Autodesk Inventor part; units mm, degrees
ref_plane "YZ Plane" through (0, 0, 0) normal (1, 0, 0) x (0, 1, 0)
ref_plane "XZ Plane" through (0, 0, 0) normal (0, 1, 0) x (-1, 0, 0)
ref_plane "XY Plane" through (0, 0, 0) normal (0, 0, 1) x (1, 0, 0)
sketch "Sketch1" plane through (0, 0, 0) normal (0, 0, 1) x (1, 0, 0)
  circle A0 centre (0, 0) radius 80
  dimension "d0" = 160
extrude "Extrusion1" add sketch "Sketch1" along normal blind 27.5
sketch "Sketch2" plane through (0, 0, 27.5) normal (0, 0, 1) x (1, 0, 0)
  circle A0 centre (0, 0) radius 70
  dimension "d3" = 140
extrude "Extrusion2" cut sketch "Sketch2" against normal blind 20
fillet "Fillet3" radius 12.5 1 edges at (-70, 0, 7.5)
fillet "Fillet4" radius 27.5 1 edges at (-80, 0, 0)
sketch "Sketch4" plane through (0, 0, 7.5) normal (0, 0, 1) x (1, 0, 0)
  circle A0 centre (0, 0) radius 21
  dimension "d13" = 42
extrude "Extrusion4" add sketch "Sketch4" along normal blind 8
sketch "Sketch6" plane through (0, 0, 27.5) normal (0, 0, 1) x (1, 0, 0)
  point P0 (0, 0)
  point P1 (0, 75)
  point P2 (75, 0)
  point P3 (0, -75)
  point P4 (-75, 0)
  dimension "d24" = 75
  dimension "d25" = 75
  dimension "d26" = 75
hole "Hole2" at (0, 75, 27.5) at (75, 0, 27.5) at (0, -75, 27.5) at (-75, 0, 27.5) direction (0, 0, -1) diameter 3.242 depth 10
sketch "Sketch8" plane through (0, 0, 15.5) normal (0, 0, 1) x (1, 0, 0)
  point P0 (0, 0)
  point P1 (0, 0)
hole "Hole4" at (0, 0, 15.5) direction (0, 0, -1) diameter 3.5 end through all
sketch "Sketch9" plane through (0, 0, 0) normal (0, 0, -1) x (-1, 0, 0)
  circle A0 centre (0, 0) radius 1.75
  circle A1 centre (0, 0) radius 19
  dimension "d56" = 38
extrude "Extrusion5" cut sketch "Sketch9" against normal blind 9
sketch "Sketch10" plane through (0, 0, 9) normal (0, 0, -1) x (-1, 0, 0)
  circle A0 centre (0, 0) radius 1.75
  circle A1 centre (0, 0) radius 6.75
  dimension "d59" = 13.5
extrude "Extrusion6" cut sketch "Sketch10" against normal blind 4.6
sketch "Sketch11" plane through (0, 0, 15.5) normal (0, 0, 1) x (1, 0, 0)
  point P0 (0, 0)
  point P1 (12.5, 0)
  point P2 (-12.5, 0)
  dimension "d74" = 12.5
  dimension "d75" = 12.5
hole "Hole5" at (12.5, 0, 15.5) at (-12.5, 0, 15.5) direction (0, 0, -1) diameter 3.2 end through all counterbore diameter 6 counterbore depth 3.2
sketch "Sketch13" plane through (0, 0, 7.5) normal (0, 0, 1) x (1, 0, 0)
  circle A0 centre (0, 0) radius 21
  line L0 (12.5, -16.8745) -> (12.5, -23.249)
  line L1 (12.5, -23.249) -> (-12.5, -23.249)
  line L2 (-12.5, -23.249) -> (-12.5, -16.8745)
  dimension "d88" = 25
  dimension "d89" = 12.5
extrude "Extrusion7" add sketch "Sketch13" along normal blind 8 contours A0 L0 L1 L2
sketch "Sketch18" plane through (0, 0, 15.5) normal (0, 0, 1) x (1, 0, 0)
  point P0 (0, 0)
  point P1 (11.3, -14.5)
  point P2 (-11.3, -14.5)
  dimension "d119" = 14.5
  dimension "d120" = 11.3
  dimension "d121" = 11.3
  dimension "d122" = 14.5
hole "Hole8" at (11.3, -14.5, 15.5) at (-11.3, -14.5, 15.5) direction (0, 0, -1) diameter 1.567 depth 5
sketch "Sketch20" plane through (0, 0, 15.5) normal (0, 0, 1) x (1, 0, 0)
  line L0 (9.25, -9.249) -> (-9.25, -9.249)
  line L1 (-9.25, -9.249) -> (-9.25, -20.249)
  line L2 (-9.25, -20.249) -> (9.25, -20.249)
  line L3 (9.25, -20.249) -> (9.25, -9.249)
  line L4 (-12.5, -23.249) -> (12.5, -23.249)
  circle A0 centre (11.3, -14.5) radius 0.7835
  point P0 (0, 0)
  dimension "d141" = 14
  dimension "d142" = 3
  dimension "d171" = 9.25
  dimension "d172" = 9.25
extrude "Extrusion12" cut sketch "Sketch20" against normal blind 17 contours L3 L2 L1 L0
fillet "Fillet10" radius 3 4 edges at (9.25, -9.249, 12.25) (9.25, -20.249, 7.75) (-9.25, -9.249, 12.25) (-9.25, -20.249, 7.75)
fillet "Fillet11" radius 3 4 edges at (12.5, -16.8745, 11.5) (12.5, -23.249, 11.5) (-12.5, -23.249, 11.5) (-12.5, -16.8745, 11.5)
chamfer "Chamfer2" distance 0.25 angle 45 4 edges at (0, 21, 15.5) (-12.5, -19.2862, 15.5) (0, -23.249, 15.5) (12.5, -19.2862, 15.5)
sketch "Sketch21" plane through (0, 0, 7.5) normal (0, 0, 1) x (1, 0, 0)
  circle A0 centre (0, 0) radius 1.75
  circle A1 centre (-40, -20) radius 4
  circle A2 centre (-40, 20) radius 4
  circle A3 centre (40, -20) radius 4
  circle A4 centre (40, 20) radius 4
  dimension "d147" = 40
  dimension "d148" = 20
  dimension "d149" = 20
  dimension "d150" = 20
  dimension "d151" = 20
  dimension "d152" = 40
  dimension "d153" = 40
  dimension "d154" = 40
  dimension "d155" = 8
  dimension "d156" = 8
  dimension "d157" = 8
  dimension "d158" = 8
extrude "Extrusion13" add sketch "Sketch21" along normal blind 3 contours A1 | A2 | A3 | A4
sketch "Sketch22" plane through (-40, 20, 10.5) normal (0, 0, 1) x (1, 0, 0)
  circle A0 centre (0, -40) radius 4
  circle A1 centre (80, 0) radius 4
  circle A2 centre (80, -40) radius 4
  point P0 (40, -20)
  point P1 (0, 0)
hole "Hole9" at (-40, -20, 10.5) at (-40, 20, 10.5) at (40, 20, 10.5) at (40, -20, 10.5) direction (0, 0, -1) diameter 3 end through all counterbore diameter 6 counterbore depth 3.2
chamfer "Chamfer3" distance 0.2 angle 45 19 edges at (36, -20, 10.5) (-44, -20, 10.5) (-44, 20, 10.5) (36, 20, 10.5) (-40, -17, 10.5) (40, -17, 10.5) (-40, 23, 10.5) (40, 23, 10.5) (8.3713, -10.1276, 15.5) (0, -9.249, 15.5) (-8.3713, -10.1276, 15.5) (-9.25, -14.749, 15.5) (-8.3713, -19.3703, 15.5) (0, -20.249, 15.5) (8.3713, -19.3703, 15.5) (9.25, -14.749, 15.5) (0, 1.75, 15.5) (-12.5, 3, 15.5) (12.5, 3, 15.5)
chamfer "Chamfer5" distance 1 angle 45 6 edges at (0, 19, 0) (0, -20.249, 0) (8.3713, -19.3703, 0) (9.25, -16.9226, 0) (-8.3713, -19.3703, 0) (-9.25, -16.9226, 0)
chamfer "Chamfer6" distance 0.5 angle 45 3 edges at (-70, 0, 27.5) (-80, 0, 27.4995) (-80, 0, 27.5)
properties part number "bottom cover" material "Aluminum 6061"
Work out the finished part from the listing and answer in its coordinate system (mm). A direction names the side the tool comes from. Give positions to 0.01 mm unless a question says otherwise; leave off trailing zeros. Answer as CSV lines item,"result".
Q1. Find the intervals of material crossed by probe 1 along X at (y, z) = (-14.5, 15); probe 2 along Y at (x, z) = (-11.3, 12.5); probe 3 along X at (y, z) = (-20, 3.5), in increasing order. Write a range as [from, to].
A:
probe 1,"x = [-75.62, -67.41], [-15.19, -12.08], [-10.52, -9.25], [9.25, 10.52], [12.08, 15.19], [67.41, 75.62]"
probe 2,"y = [-74.7, -66.55], [-22.65, -15.28], [-13.72, -2.75], [2.75, 17.7], [66.55, 74.7]"
probe 3,"x = [-62.82, -41.5], [-38.5, -7.45], [7.45, 38.5], [41.5, 62.82]"
Q2. A tool of negligible diameter and unlimited length cuts with its end or side. For faces 3 (the cylindrical face through (37.97, 22.21, 8.78)), 4 (the flat face through (9.25, -15, 11)), 5 (the cylindrical face through (1.46, -6.59, 11.27)), from which of +Z, -Z, +X, -X, +Y, -Y can it reach the whole face along a straight path? Write none if from no direction.
A:
face 3,"+Z"
face 4,"+Z, -Z"
face 5,"-Z"
Q3. Given P1, Ø10, axis at y = -15.5, z = 23.5, coming from the -X side; P2, Ø15, axis at x = 1, y = -2.5, coming from the -Z side; P3, Ø9.5, axis at x = 40, y = 20, coming from the +Z side, each flat-ended and moving along its own axis, determine where each tip first touches the part or whether it passes through.
A:
P1,"stops at x = -79.18"
P2,"stops at z = 9"
P3,"stops at z = 10.5"
Q4. The mould has two halves that part along X. Classify faces 1 (the flat face through (23, 1, 0)), 2 (the flat face through (0, -20.249, 8)): +X half, -X half, draft (parallel to the pull), parting line (faces both ways), or undercut.
A:
face 1,"draft"
face 2,"undercut"
